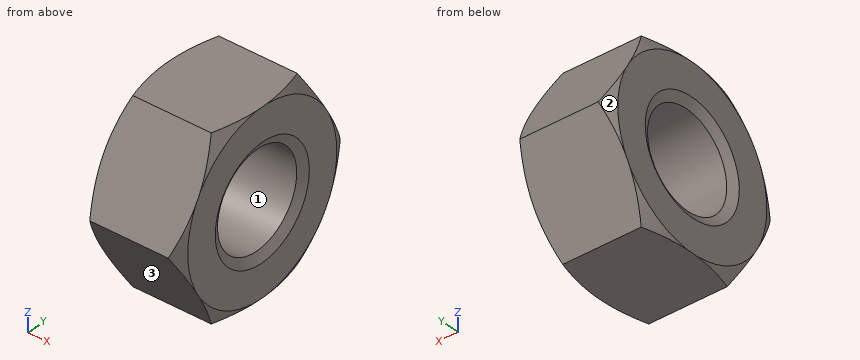
Autodesk Inventor part; units mm, degrees
ref_plane "Work Plane1" through (-20.6974, 0, 0) normal (0, -0.866, -0.5) x (1, 0, 0)
ref_plane "YZ Plane" through (0, 0, 0) normal (1, 0, 0) x (0, 1, 0)
ref_plane "XZ Plane" through (0, 0, 0) normal (0, 1, 0) x (-1, 0, 0)
sketch "Эскиз1" plane through (0, 0, 0) normal (1, 0, 0) x (0, 1, 0)
  line L0 (-10.9697, 0) -> (-5.4848, 9.5)
  line L1 (-5.4848, 9.5) -> (5.4848, 9.5)
  line L2 (5.4848, 9.5) -> (10.9697, 0)
  line L3 (10.9697, 0) -> (5.4848, -9.5)
  line L4 (5.4848, -9.5) -> (-5.4848, -9.5)
  line L5 (-5.4848, -9.5) -> (-10.9697, 0)
  point P0 (0, 0)
  point P1 (0, 0)
  dimension "d0" = 21.9393
extrude "Базовый элемент" add sketch "Эскиз1" along normal blind 10
sketch "Эскиз2" plane through (0, 0, 0) normal (0, 0, 1) x (1, 0, 0)
  line L0 (0, 5.4848) -> (0, 10.9697)
  line L1 (0, 10.9697) -> (10, 10.9697)
  line L2 (10, 5.4848) -> (10, 10.9697)
  line L3 (-2, 0) -> (12, 0)
  line L4 (0.8485, 10.9697) -> (0, 9.5)
  line L5 (9.1515, 10.9697) -> (10, 9.5)
  dimension "d3" = 30
  dimension "d4" = 30
  dimension "d5" = 19
  dimension "d6" = 19
revolve "Фаска1" cut sketch "Эскиз2" angle 360 about axis through (-10, 0, 0) along (1, 0, 0)
sketch "Эскиз3" plane through (10, 0, 0) normal (1, 0, 0) x (0, 0, -1)
  arc A0 (-4.75, -8.2272) -> (4.75, -8.2272) centre (0, 0) ccw
hole "Резьба" at (10, 0, 0) direction (-1, 0, 0) diameter 10.106 end through all
chamfer "Фаска2" distance 0.9472 angle 30 1 edges at (10, 0, 5.053) measured on face at (10, -7.9707, -0.203)
chamfer "Фаска3" distance 0.9472 angle 30 1 edges at (0, 0, 5.053) measured on face at (0, -7.9707, -0.203)
ref_plane "Work Plane1" through (-20.6974, 0, 0) normal (0, -0.866, -0.5) x (1, 0, 0)
equation "\"d0\" = 1.1547 * SW"
equation "\"d1\" = KOH"
equation "\"d3\" = ANG1"
equation "\"d4\" = ANG2"
equation "\"d5\" = SW0"
equation "\"d6\" = SW01"
equation "\"d8\" = -0.5 * GD1 + 0.5 * NND"
equation "\"d40\" = -0.5 * GD1 + 0.5 * NND"
equation "\"d10\" = -0.5 * GD1 + 0.5 * NND"
equation "\"d41\" = -0.5 * GD1 + 0.5 * NND"
equation "\"ANG1\" = 30deg"
equation "\"ANG2\" = 30deg"
equation "\"NND\" = 12"
equation "\"KOH\" = 10"
equation "\"SW\" = 19"
equation "\"SW0\" = 19"
equation "\"SW01\" = SW0"
equation "\"GUL\" = 0.541266 * PTC"
equation "\"LADI\" = 18.05"
equation "\"TOA\" = 30deg"
equation "\"FAWI\" = 30deg"
equation "\"PTC\" = 1.75"
equation "\"THREADDIA\" = 12"
equation "\"E0\" = 1.155 * SW"
equation "\"GAL\" = 0.541266 * PTC"
properties part number "Гайка M12-6H ГОСТ 5927-70" material "Сталь, мягкая"
Verification items for the finished model (mm, model axes). Face numbers are marked on the shaded views. Coordinates: 2 decimals unless noted, no trailing zeros. Loops run counter-clockwise (first coordinate to the right, second up) from the corner with the lowest first, then second, coordinate; pieces in that order, holes last. Notation, with made-up numbers: (16, 78.25) -> (61, 78.25) arc R13 cw to (61, 103.25) -> close; hole circle Ø4 at (28, 25). An arc over 180 degrees is marked (long way). Write each question's results on one line, items separated by ' | '.
Item 1: Mould release check, pull along Z, two halves, no side actions. Record for the marked faces 1, 2 and 3: +Z half, -Z half, draft (parallel to the pull), parting line (faces both ways), or undercut.
Found:
face 1: undercut | face 2: parting line | face 3: -Z half
Item 2: Gauge pin test, flat ends, axial feed: pin 1 (2 mm diameter, centred on x = 8, y = -7.5, fed in from -Z); pin 2 (1.5 mm diameter, centred on x = 1.5, z = 2, fed in from -Y); pin 3 (9 mm diameter, centred on y = 0, z = 0, fed in from +X); pin 4 (1.5 mm diameter, centred on x = 2, z = 6, fed in from +Y). Record the tip position at first contact, or that the pin passes through.
Found:
pin 1: stops at z = -7.74 | pin 2: stops at y = -10.25 | pin 3: passes through | pin 4: stops at y = 7.94
Item 3: Section check A-A, the plane x = 8.5. Enter the section's corners in (y, z).
Found:
outline: (-10.97, 0) -> (-5.48, -9.5) -> (5.48, -9.5) -> (10.97, 0) -> (5.48, 9.5) -> (-5.48, 9.5) -> close; hole circle Ø10.11 at (0, 0)
Item 4: Material ranges on L1, parallel to Z at x = 4.5, y = 0; L2, parallel to Y at x = 4.25, z = -3, recorded low to high.
Found:
L1: z = -9.5 to -5.05, 5.05 to 9.5 | L2: y = -9.24 to -4.07, 4.07 to 9.24
